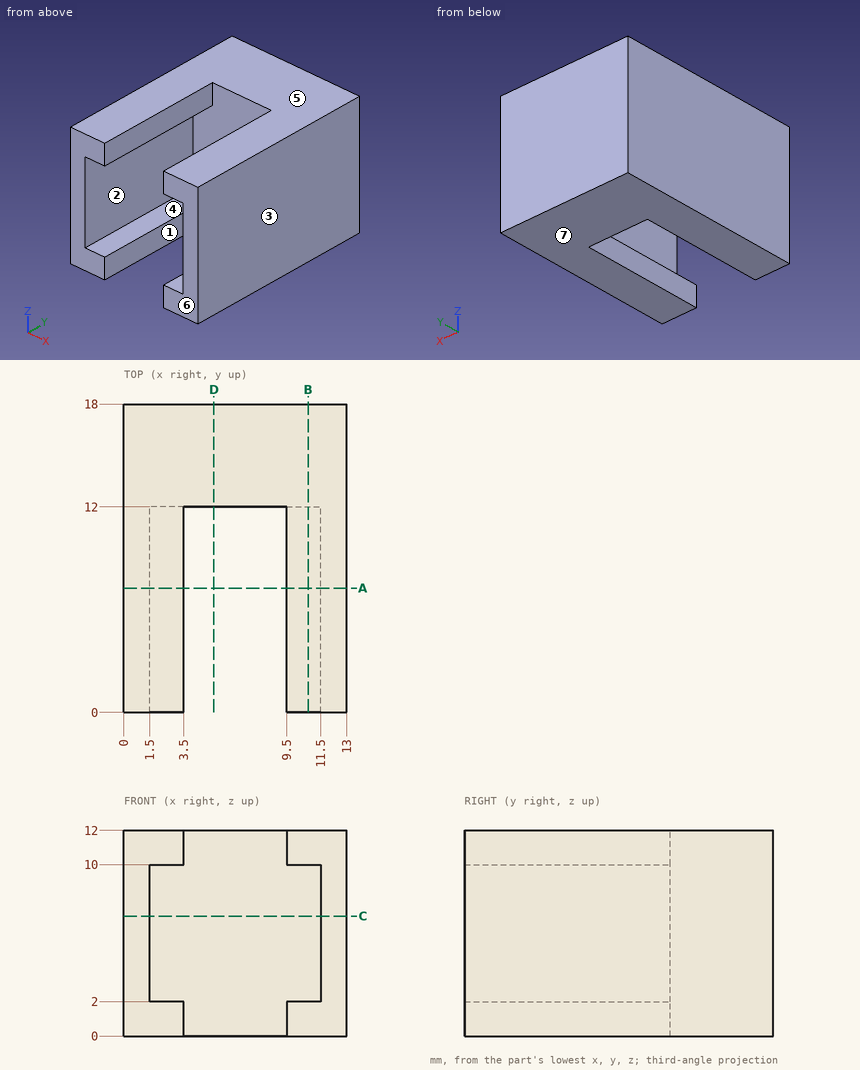
Study the drawing (mm; zero at the part's minimum x, y, z) and answer. A direction names the side the tool comes from. Coordinates: 2 decimals unless noted, no trailing zeros. Write each loop counter-clockwise with the first axis right and the second up, starting at its lowest first coordinate (ties: lowest second). Pieces come first, ordered by that corner, then holes. Notation, with made-up numbers: M 84,72 L 102,72 A8 cw 102,76 Z; hole C 65.25,33 d1. An arc over 180 degrees is marked long. Use a Markdown table: item, result. Add a question column.
1. Straight lines are drawn through the part: line 1 along X through (y, z) = (8.5, 3.5); line 2 along Y through (x, z) = (3, 3.25); line 3 along Z through (x, y) = (2, 5.5). For each, find the intervals that lie inside material, in ascending order. Write a range as [from, to].
2. Section B-B (x = 10.75) is taken. Give the vertices of the cut face in (y, z), plus the area to 3 significant figures.
3. For a pull along Z with two mould halves and no side action, classify the marked faces 4, 5, 6 and 7 as +Z half, -Z half, draft (parallel to the pull), parting line (faces both ways), or undercut.
4. Section D-D (x = 5.25) is taken. Give the vertices of the cut face in (y, z).
5. Given P1, Ø2.5, axis at y = 6, z = 5, coming from the -X side, flat-ended and moving along its own axis, determine where the tip first touches the part or whether it passes through.
6. Section C-C (z = 7) is taken. Give the vertices of the cut face in (x, y), plus the area to 3 significant figures.
7. Section A-A (y = 7.25) is taken. Give the vertices of the cut face in (x, z), plus the area to 3 significant figures.
8. Which of the six approach directions +Z, -Z, +X, -X, +Y, -Y give full straight-line access (tool end or side, diameter ignored) to the marked faces 1, 2 and 3?
Data:
| question | item | result |
|---|---|---|
| 1 | line 1 | x = [0, 1.5], [11.5, 13] |
| 1 | line 2 | y = [12, 18] |
| 1 | line 3 | z = [0, 2], [10, 12] |
| 2 | outline | M 0,0 L 18,0 L 18,12 L 0,12 L 0,10 L 12,10 L 12,2 L 0,2 Z |
| 2 | area | 120 mm2 |
| 3 | face 4 | undercut |
| 3 | face 5 | +Z half |
| 3 | face 6 | draft |
| 3 | face 7 | -Z half |
| 4 | outline | M 12,0 L 18,0 L 18,12 L 12,12 Z |
| 5 | P1 | stops at x = 0 |
| 6 | outline | M 0,0 L 1.5,0 L 1.5,12 L 11.5,12 L 11.5,0 L 13,0 L 13,18 L 0,18 Z |
| 6 | area | 114 mm2 |
| 7 | outline | M 0,0 L 3.5,0 L 3.5,2 L 1.5,2 L 1.5,10 L 3.5,10 L 3.5,12 L 0,12 Z; M 9.5,0 L 13,0 L 13,12 L 9.5,12 L 9.5,10 L 11.5,10 L 11.5,2 L 9.5,2 Z |
| 7 | area | 52.0 mm2 |
| 8 | face 1 | +Z, -Z, -Y |
| 8 | face 2 | -Y |
| 8 | face 3 | +Z, -Z, +X, +Y, -Y |
